```python
from build123d import *

# Parameters (mm, degrees)
BOSS_EXTRUDE1_DEPTH = 19.05
SKETCH2_R           = 5.55625
CUT_EXTRUDE1_DEPTH  = 8.1755
SKETCH3_R           = 3.3782
CUT_EXTRUDE2_DEPTH  = 4.175


with BuildPart() as part:
    # Sketch1 → Boss-Extrude1 (new body)
    with BuildSketch(Plane.XY):
        Polygon((-76.2, 0), (76.2, 0), (76.2, 3.175), (63.5, 3.175), (63.5, 7.1755), (-63.5, 7.1755), (-63.5, 3.175), (-76.2, 3.175), align=None)
    extrude(amount=BOSS_EXTRUDE1_DEPTH)

    # Sketch2 → Cut-Extrude1 (cut, through all)
    with BuildSketch(Plane(origin=(0, 7.1755, 0), x_dir=(1, 0, 0), z_dir=(0, 1, 0))):
        with Locations((0, -9.525)):
            Circle(SKETCH2_R)
    extrude(amount=-CUT_EXTRUDE1_DEPTH, mode=Mode.SUBTRACT)

    # Sketch3 → Cut-Extrude2 (cut, through all)
    with BuildSketch(Plane(origin=(0, 3.175, 0), x_dir=(1, 0, 0), z_dir=(0, 1, 0))):
        with Locations((-69.85, -9.525)):
            Circle(SKETCH3_R)
        with Locations((69.85, -9.525)):
            Circle(SKETCH3_R)
    extrude(amount=-CUT_EXTRUDE2_DEPTH, mode=Mode.SUBTRACT)


solid = part.part
```
Check sheet for the modelled part. Datum: model origin and axes. Units: mm. A direction names the side the tool comes from. Give positions to 0.01 mm unless a question says otherwise; leave off trailing zeros. Order: outer loops, then holes, each group sorted by start corner. A loop starts at its lowest first (then second) coordinate and runs counter-clockwise, first axis right, second up. Notation, with made-up numbers: (8.5, -12) -> (67.5, -12) arc R8 ccw to (67.5, -2) -> close; hole circle Ø3 at (44, 56). An arc over 180 degrees is marked (long way). Use CSV: the item, a comma, the result in double quotes. Start each with the question number.
1) Sectioned sample at B-B, the plane x = 69.85. Record the boundary of the cut face in (y, z) (3 decimals).
2) Sectioned sample at A-A, the plane x = 0. Record the boundary of the cut face in (y, z).
3) Material ranges on line 1 (X direction, y = 2, z = 10.5); line 2 (Z direction, x = 69.85, y = 2.4); line 3 (X direction, y = 2.5, z = 9), recorded low to high. Write a range as from..to.
4) Set-up check for faces 4 (the face through (-63.5, 5, 9)), 5 (the face through (66.475, 1.61, 9.376)), 6 (the face through (73, 3.175, 7)): record each of +Z, -Z, +X, -X, +Y, -Y from which the full face is reachable in a straight line by a thin tool's end or side.
5) Mould release check, pull along Z, two halves, no side actions. Record for faces 1 (the face through (-1, 4, 0)), 2 (the face through (1, 7.176, 16)), 3 (the face through (-0.723, 3.638, 4.016)): released by +Z, released by -Z, zero draft, split by the parting line, or undercut.
6) Sectioned sample at D-D, the plane z = 2. Record the boundary of the cut face in (x, y) (1 decimal), plus the area to 3 significant figures.
7) Go/stop test with flat-tipped pins: P1, Ø10, axis at x = -69, z = 14, coming from the +Y side (3 decimals); P2, Ø2, axis at y = 6, z = 13, coming from the +X side; P3, Ø10, axis at x = 0, z = 9.525, coming from the -Y side. Record where each tip stops, or that it passes through.
Recorded:
1,outline,"(0, 0) -> (3.175, 0) -> (3.175, 6.147) -> (0, 6.147) -> close; (0, 12.903) -> (3.175, 12.903) -> (3.175, 19.05) -> (0, 19.05) -> close"
2,outline,"(0, 0) -> (7.18, 0) -> (7.18, 3.97) -> (0, 3.97) -> close; (0, 15.08) -> (7.18, 15.08) -> (7.18, 19.05) -> (0, 19.05) -> close"
3,line 1,"-76.2..-73.08, -66.62..-5.47, 5.47..66.62, 73.08..76.2"
3,line 2,"0..6.15, 12.9..19.05"
3,line 3,"-76.2..-73.19, -66.51..-5.53, 5.53..66.51, 73.19..76.2"
4,face 4,"+Z, -Z, -X, +Y"
4,face 5,"+Y, -Y"
4,face 6,"+Z, -Z, +X, +Y"
5,face 1,"released by -Z"
5,face 2,"zero draft"
5,face 3,"undercut"
6,outline,"(-76.2, 0) -> (76.2, 0) -> (76.2, 3.2) -> (63.5, 3.2) -> (63.5, 7.2) -> (-63.5, 7.2) -> (-63.5, 3.2) -> (-76.2, 3.2) -> close"
6,area,"992 mm2"
7,P1,"y = 3.175"
7,P2,"x = 63.5"
7,P3,"through"
